The model under review builds one solid part; all positions refer to its coordinate system, in mm. A direction names the side the tool comes from. Coordinates: 2 decimals unless noted, no trailing zeros. Write each loop counter-clockwise with the first axis right and the second up, starting at its lowest first coordinate (ties: lowest second). Pieces come first, ordered by that corner, then holes. Notation, with made-up numbers: (1.25, 88) -> (6.25, 88) arc R21 cw to (6.25, 112) -> close; hole circle Ø8 at (77, 7). An arc over 180 degrees is marked (long way). Put each result on its own line as item: value. Start each with the question number.
from build123d import *

# Parameters (mm, degrees)
EXTRUDE_1_DEPTH     = 4
EXTRUDE_2_DEPTH     = 4
FILLET_1_R          = 10
CUT_EXTRUDE_1_DEPTH = 142.340015565
SKETCH_4_W          = 6
SKETCH_4_H          = 6
EXTRUDE_7_DEPTH     = 4
SKETCH_6_R          = 1.5
CUT_EXTRUDE_4_DEPTH = 142.774468788
CUT_EXTRUDE_5_DEPTH = 142.774468788
FILLET_5_R          = 1
FILLET_6_R          = 1


with BuildPart() as part:
    # Эскиз1 → Бобышка-Вытянуть1 (new body)
    with BuildSketch(Plane(origin=(0, 0, 0), x_dir=(1, 0, 0), z_dir=(0, 1, 0))):
        Polygon((-140, -17), (-140, 17), (-138, 19), (-132, 19), (-132, 8), (0, 8), (0, -8), (-132, -8), (-132, -19), (-138, -19), align=None)
    extrude(amount=EXTRUDE_1_DEPTH)

    # Эскиз2 → Бобышка-Вытянуть2 (add)
    # profile 1 of 2: a face of its own
    with BuildSketch(Plane.XZ):
        with BuildLine():
            Line((-63, 16), (-5, 16))
            ThreePointArc((-5, 16), (0, 11), (-5, 6))
            Line((-5, 6), (-63, 6))
            ThreePointArc((-63, 6), (-68, 11), (-63, 16))
        make_face()
        with BuildLine():
            Line((-63, 13), (-5, 13))
            ThreePointArc((-5, 13), (-3, 11), (-5, 9))
            Line((-5, 9), (-63, 9))
            ThreePointArc((-63, 9), (-65, 11), (-63, 13))
        make_face(mode=Mode.SUBTRACT)
    # profile 2 of 2: a face of its own
    with BuildSketch(Plane.XZ):
        with BuildLine():
            Line((-63, -16), (-5, -16))
            ThreePointArc((-5, -16), (0, -11), (-5, -6))
            Line((-5, -6), (-63, -6))
            ThreePointArc((-63, -6), (-68, -11), (-63, -16))
        make_face()
        with BuildLine():
            Line((-63, -13), (-5, -13))
            ThreePointArc((-5, -13), (-3, -11), (-5, -9))
            Line((-5, -9), (-63, -9))
            ThreePointArc((-63, -9), (-65, -11), (-63, -13))
        make_face(mode=Mode.SUBTRACT)
    extrude(amount=-EXTRUDE_2_DEPTH)

    # Скругление1
    # the kernel refuses this fillet: 10 mm, written as the material it adds along each edge
    with BuildSketch(Plane(origin=(-1, 4, 8), x_dir=(1, 0, 0), z_dir=(0, -1, 0))) as fillet_1_piece_1:
        with BuildLine():
            CenterArc((10.90874153, 1.347902551), FILLET_1_R, 173.676623786, 14.069867748)
            Line((0.96958051, 2.44930085), (0.77079729, 2.471328816))
            ThreePointArc((0.77079729, 2.471328816), (0.463030841, 1.233264109), (-0.16, 0.12))
            Line((-0.16, 0.12), (0, -0.2))
            ThreePointArc((0, -0.2), (0.5, -0.2), (0.801825169, -0.026958051))
            Line((0.801825169, -0.026958051), (1, 0))
        make_face()
    extrude(amount=4)
    with BuildSketch(Plane(origin=(-67, 4, 8), x_dir=(-1, 0, 0), z_dir=(0, -1, 0))) as fillet_1_piece_2:
        with BuildLine():
            CenterArc((9.266499161, -10), FILLET_1_R, 90, 62.181860715)
            Line((0.422166387, -5.333333333), (0.245279732, -5.24))
            ThreePointArc((0.245279732, -5.24), (0.785032611, -2.621235013), (-0.16, -0.12))
            Line((-0.16, -0.12), (0, 0.2))
            Line((0, 0.2), (9.266499161, 0.2))
            Line((9.266499161, 0.2), (9.266499161, 0))
        make_face()
    extrude(amount=4)
    with BuildSketch(Plane(origin=(-1, 4, -8), x_dir=(1, 0, 0), z_dir=(0, -1, 0))) as fillet_1_piece_3:
        with BuildLine():
            CenterArc((10.90874153, -1.347902551), FILLET_1_R, 172.253508466, 14.069867748)
            Line((0.96958051, -2.44930085), (0.77079729, -2.471328816))
            ThreePointArc((0.77079729, -2.471328816), (0.463030841, -1.233264109), (-0.16, -0.12))
            Line((-0.16, -0.12), (0, 0.2))
            ThreePointArc((0, 0.2), (0.5, 0.2), (0.801825169, 0.026958051))
            Line((0.801825169, 0.026958051), (1, 0))
        make_face()
    extrude(amount=4)
    with BuildSketch(Plane(origin=(-67, 4, -8), x_dir=(-1, 0, 0), z_dir=(0, -1, 0))) as fillet_1_piece_4:
        with BuildLine():
            CenterArc((9.266499161, 10), FILLET_1_R, 207.818139285, 62.181860715)
            Line((0.422166387, 5.333333333), (0.245279732, 5.24))
            ThreePointArc((0.245279732, 5.24), (0.785032611, 2.621235013), (-0.16, 0.12))
            Line((-0.16, 0.12), (0, -0.2))
            Line((0, -0.2), (9.266499161, -0.2))
            Line((9.266499161, -0.2), (9.266499161, 0))
        make_face()
    extrude(amount=4)

    # Эскиз3 → Вырез-Вытянуть1 (cut, through all)
    with BuildSketch(Plane.XZ):
        with BuildLine():
            Line((-24.36067626, 3.753765504), (-128.863745401, 3.753765504))
            ThreePointArc((-128.863745401, 3.753765504), (-132.613745401, 0.003765504), (-128.863745401, -3.746234496))
            Line((-128.863745401, -3.746234496), (-24.36067626, -3.746234496))
            ThreePointArc((-24.36067626, -3.746234496), (-20.61067626, 0.003765504), (-24.36067626, 3.753765504))
        make_face()
    extrude(amount=-CUT_EXTRUDE_1_DEPTH, mode=Mode.SUBTRACT)

    # Эскиз4 → Бобышка-Вытянуть7 (add)
    with BuildSketch(Plane(origin=(0, 4, 0), x_dir=(1, 0, 0), z_dir=(0, 1, 0))):
        with Locations((-24, -19)):
            Rectangle(SKETCH_4_W, SKETCH_4_H)
    extrude(amount=-EXTRUDE_7_DEPTH)

    # Эскиз6 → Вырез-Вытянуть4 (cut, through all)
    with BuildSketch(Plane(origin=(0, 4, 0), x_dir=(1, 0, 0), z_dir=(0, 1, 0))):
        with Locations(Location((-24, -19, 0), (0, 0, 270))):
            Circle(SKETCH_6_R)
    extrude(amount=-CUT_EXTRUDE_4_DEPTH, mode=Mode.SUBTRACT)

    # Эскиз7 → Вырез-Вытянуть5 (cut, through all)
    with BuildSketch(Plane(origin=(0, 4, 0), x_dir=(1, 0, 0), z_dir=(0, 1, 0))):
        Polygon((-140, 16.36754244), (-131.974442882, 18.073427267), (-132, 19), (-138, 19), (-140, 17), align=None)
    cut_extrude_5 = extrude(amount=-CUT_EXTRUDE_5_DEPTH, mode=Mode.SUBTRACT)

    # Скругление5
    fillet_5_edges = [part.edges().sort_by_distance(p)[0] for p in [
        (-140, 2, -16.36754244),
    ]]
    fillet(fillet_5_edges, radius=FILLET_5_R)

    # Зеркальное отражение5: Вырез-Вытянуть5 across plane
    add(cut_extrude_5.mirror(Plane.XY), mode=Mode.SUBTRACT)

    # Скругление6
    fillet_6_edges = [part.edges().sort_by_distance(p)[0] for p in [
        (-140, 2, 16.36754244),
    ]]
    fillet(fillet_6_edges, radius=FILLET_6_R)


solid = part.part
1. Consider section B-B on z = 0. State the section outline as (x, y) points, then the cut area to 3 significant figures.
2. Tool access review of faces 5 (the flat face through (-21, 2, 19)), 6 (the cylindrical face through (-66, 2, -15)), 7 (the flat face through (-34, 2, -9)), 8 (the flat face through (-45, 2, 16)): name each direction out of +Z, -Z, +X, -X, +Y, -Y from which nothing blocks a thin tool from reaching the whole face with its end or side.
3. Wall thickness on line 1 (Z direction, x = -55.5, y = 3.6); line 2 (X direction, y = 0.85, z = 19); line 3 (X direction, y = 2.8, z = -11): over which ranges is each line inside the solid? List them lowest first. Write a range as from..to.
4. The part is to be moulded in two halves that separate along X. For faces 1 (the cylindrical face through (-0.09, 2.03, 9.24)), 2 (the flat face through (-105, 2, -8)), 3 (the flat face through (-71, 0, 6)), 4 (the flat face through (-104, 2, 8)), say which applies: released by +X, released by -X, zero draft, split by the parting line, or undercut.
5. Consider section A-A on x = -36. State the section outline as (y, z) points, then the cut area to 3 significant figures.
6. Consider section D-D on x = -18.5. State the section outline as (y, z) points.
7. Consider section C-C on x = -122.5. State the section outline as (y, z) points, then the cut area to 3 significant figures.
8. Insertion check: P1, Ø1, axis at y = 3, z = 16.5, coming from the -X side; P2, Ø2.5, axis at x = -24, z = 19, coming from the +Y side; P3, Ø2, axis at x = -108, y = 2.5, coming from the +Z side; P4, Ø2, axis at x = -41, y = 2, coming from the +Z side. Each pin has a flat end and moves straight along its axis. Give the tip position at first contact, or say it passes through.
Output values:
1. outline: (-140, 0) -> (-132.61, 0) -> (-132.61, 4) -> (-140, 4) -> close; (-20.61, 0) -> (0, 0) -> (0, 4) -> (-20.61, 4) -> close
1. area: 112 mm^2
2. face 5: +Z, +X, +Y, -Y
2. face 6: -Z, +Y, -Y
2. face 7: +Y, -Y
2. face 8: +Z, +Y, -Y
3. line 1: z = -16..-13, -9..-3.75, 3.75..9, 13..16
3. line 2: x = -27..-25.5, -22.5..-21
3. line 3: x = -140..-132, -69.13..-65, -3..0
4. face 1: released by +X
4. face 2: undercut
4. face 3: zero draft
4. face 4: undercut
5. outline: (0, -16) -> (4, -16) -> (4, -13) -> (0, -13) -> close; (0, -9) -> (4, -9) -> (4, -3.75) -> (0, -3.75) -> close; (0, 3.75) -> (4, 3.75) -> (4, 9) -> (0, 9) -> close; (0, 13) -> (4, 13) -> (4, 16) -> (0, 16) -> close
5. area: 66.0 mm^2
6. outline: (0, -16) -> (4, -16) -> (4, -13) -> (0, -13) -> close; (0, -9) -> (4, -9) -> (4, 9) -> (0, 9) -> close; (0, 13) -> (4, 13) -> (4, 16) -> (0, 16) -> close
7. outline: (0, -8) -> (4, -8) -> (4, -3.75) -> (0, -3.75) -> close; (0, 3.75) -> (4, 3.75) -> (4, 8) -> (0, 8) -> close
7. area: 34.0 mm^2
8. P1: stops at x = -139.9
8. P2: passes through
8. P3: stops at z = 8
8. P4: stops at z = 16
